from build123d import *

# Parameters (mm, degrees)
BOSS_EXTRUDE1_DEPTH = 20.5
SKETCH2_W           = 11
SKETCH2_H           = 11
CUT_EXTRUDE1_DEPTH  = 38.791732231
SKETCH3_W           = 30.25
SKETCH3_H           = 17.75
CUT_EXTRUDE2_DEPTH  = 0.5
CUT_EXTRUDE3_REACH  = 39.609
SKETCH4_W           = 27.25
SKETCH4_H           = 14.75
SKETCH5_W           = 2
SKETCH5_H           = 1.375
SKETCH5_W_2         = 1.375
SKETCH5_H_2         = 2
BOSS_EXTRUDE2_DEPTH = 0.75
SKETCH6_W           = 1.375
SKETCH6_H           = 2
SKETCH6_W_2         = 0.3
SKETCH6_W_3         = 2
SKETCH6_H_2         = 0.3
SKETCH6_H_3         = 1.375
BOSS_EXTRUDE3_DEPTH = 0.75
SKETCH7_W           = 8
SKETCH7_H           = 2.5
CUT_EXTRUDE4_DEPTH  = 38.609374164
CUT_EXTRUDE5_REACH  = 39.528
SKETCH8_W           = 1
SKETCH8_H           = 11


with BuildPart() as part:
    # Sketch1 → Boss-Extrude1 (new body)
    with BuildSketch(Plane(origin=(0, 0, 0), x_dir=(1, 0, 0), z_dir=(0, 1, 0))):
        with BuildLine():
            Line((-21.150314886, 2.25), (-22.947265174, 1.37195122))
            ThreePointArc((-22.947265174, 1.37195122), (-22.710349254, 0.704078714), (-22.63, 0))
            ThreePointArc((-22.63, 0), (-26.459078714, -3.044650746), (-28.562734826, 1.37195122))
            Line((-28.562734826, 1.37195122), (-30.359685114, 2.25))
            ThreePointArc((-30.359685114, 2.25), (-26.90968909, -4.993227223), (-20.63, 0))
            ThreePointArc((-20.63, 0), (-20.643812376, 0.376013393), (-20.685175052, 0.75))
            ThreePointArc((-20.685175052, 0.75), (-20.85994778, 1.517922517), (-21.150314886, 2.25))
        make_face()
        with BuildLine():
            Line((21.150314886, 2.25), (-21.150314886, 2.25))
            ThreePointArc((-21.150314886, 2.25), (-20.85994778, 1.517922517), (-20.685175052, 0.75))
            Line((-20.685175052, 0.75), (20.685175052, 0.75))
            ThreePointArc((20.685175052, 0.75), (20.85994778, 1.517922517), (21.150314886, 2.25))
        make_face()
        with BuildLine():
            Line((22.947265174, 1.37195122), (21.150314886, 2.25))
            ThreePointArc((21.150314886, 2.25), (20.85994778, 1.517922517), (20.685175052, 0.75))
            ThreePointArc((20.685175052, 0.75), (25.378986607, -5.111187624), (30.88, 0))
            ThreePointArc((30.88, 0), (30.748227223, 1.15468909), (30.359685114, 2.25))
            Line((30.359685114, 2.25), (28.562734826, 1.37195122))
            ThreePointArc((28.562734826, 1.37195122), (28.799650746, 0.704078714), (28.88, 0))
            ThreePointArc((28.88, 0), (25.050921286, -3.044650746), (22.947265174, 1.37195122))
        make_face()
        with BuildLine():
            Line((23.586331053, 2.25), (21.150314886, 2.25))
            Line((21.150314886, 2.25), (22.947265174, 1.37195122))
            ThreePointArc((22.947265174, 1.37195122), (23.22836369, 1.838949145), (23.586331053, 2.25))
        make_face()
        with BuildLine():
            Line((28.562734826, 1.37195122), (30.359685114, 2.25))
            Line((30.359685114, 2.25), (27.923668947, 2.25))
            ThreePointArc((27.923668947, 2.25), (28.28163631, 1.838949145), (28.562734826, 1.37195122))
        make_face()
        with BuildLine():
            ThreePointArc((-23.586331053, 2.25), (-23.22836369, 1.838949145), (-22.947265174, 1.37195122))
            Line((-22.947265174, 1.37195122), (-21.150314886, 2.25))
            Line((-21.150314886, 2.25), (-23.586331053, 2.25))
        make_face()
        with BuildLine():
            Line((-30.359685114, 2.25), (-28.562734826, 1.37195122))
            ThreePointArc((-28.562734826, 1.37195122), (-28.28163631, 1.838949145), (-27.923668947, 2.25))
            Line((-27.923668947, 2.25), (-30.359685114, 2.25))
        make_face()
    extrude(amount=BOSS_EXTRUDE1_DEPTH)

    # Sketch2 → Cut-Extrude1 (cut, through all)
    with BuildSketch(Plane(origin=(0, 0, -2.25), x_dir=(-1, 0, 0), z_dir=(0, 0, -1))):
        with Locations((-25.38, 10.25)):
            Rectangle(SKETCH2_W, SKETCH2_H)
        with Locations((25.38, 10.25)):
            Rectangle(SKETCH2_W, SKETCH2_H)
    extrude(amount=-CUT_EXTRUDE1_DEPTH, mode=Mode.SUBTRACT)

    # Sketch3 → Cut-Extrude2 (cut)
    with BuildSketch(Plane.XY.offset(-0.75)):
        with Locations((0, 10.25)):
            Rectangle(SKETCH3_W, SKETCH3_H)
    extrude(amount=-CUT_EXTRUDE2_DEPTH, mode=Mode.SUBTRACT)

    # Sketch4 → Cut-Extrude3 (cut, up to next)
    with BuildSketch(Plane.XY.offset(-1.25), mode=Mode.PRIVATE) as cut_extrude3_sk1:
        with Locations((0, 10.25)):
            Rectangle(SKETCH4_W, SKETCH4_H)
    cut_extrude3_tool1 = extrude(cut_extrude3_sk1.sketch, amount=-CUT_EXTRUDE3_REACH, mode=Mode.PRIVATE) & part.part
    add(cut_extrude3_tool1.solids().sort_by_distance((0, 10.25, -1.25))[0], mode=Mode.SUBTRACT)

    # Sketch5 → Boss-Extrude2 (add)
    with BuildSketch(Plane.XY.offset(-0.75)):
        with Locations((0, 19.8125)):
            Rectangle(SKETCH5_W, SKETCH5_H)
        with Locations((0, 0.6875)):
            Rectangle(SKETCH5_W, SKETCH5_H)
        with Locations((-15.8125, 10.25)):
            Rectangle(SKETCH5_W_2, SKETCH5_H_2)
        with Locations((15.8125, 10.25)):
            Rectangle(SKETCH5_W_2, SKETCH5_H_2)
    extrude(amount=BOSS_EXTRUDE2_DEPTH)

    # Sketch6 → Boss-Extrude3 (add)
    with BuildSketch(Plane.XY):
        with Locations((-15.8125, 10.25)):
            Rectangle(SKETCH6_W, SKETCH6_H)
        with Locations((-14.975, 10.25)):
            Rectangle(SKETCH6_W_2, SKETCH6_H)
        with Locations((0, 1.525)):
            Rectangle(SKETCH6_W_3, SKETCH6_H_2)
        with Locations((0, 0.6875)):
            Rectangle(SKETCH6_W_3, SKETCH6_H_3)
        with Locations((14.975, 10.25)):
            Rectangle(SKETCH6_W_2, SKETCH6_H)
        with Locations((15.8125, 10.25)):
            Rectangle(SKETCH6_W, SKETCH6_H)
        with Locations((0, 19.8125)):
            Rectangle(SKETCH6_W_3, SKETCH6_H_3)
        with Locations((0, 18.975)):
            Rectangle(SKETCH6_W_3, SKETCH6_H_2)
    extrude(amount=BOSS_EXTRUDE3_DEPTH)

    # Sketch7 → Cut-Extrude4 (cut, through all)
    with BuildSketch(Plane.XY.offset(-1.25)):
        with Locations((-11.125, 17.875)):
            Rectangle(SKETCH7_W, SKETCH7_H)
    extrude(amount=-CUT_EXTRUDE4_DEPTH, mode=Mode.SUBTRACT)

    # Sketch8 → Cut-Extrude5 (cut, up to next)
    with BuildSketch(Plane.XY.offset(-0.75), mode=Mode.PRIVATE) as cut_extrude5_sk1:
        with Locations((19.38, 10.25)):
            Rectangle(SKETCH8_W, SKETCH8_H)
    cut_extrude5_tool1 = extrude(cut_extrude5_sk1.sketch, amount=-CUT_EXTRUDE5_REACH, mode=Mode.PRIVATE) & part.part
    add(cut_extrude5_tool1.solids().sort_by_distance((19.38, 10.25, -0.75))[0], mode=Mode.SUBTRACT)


solid = part.part
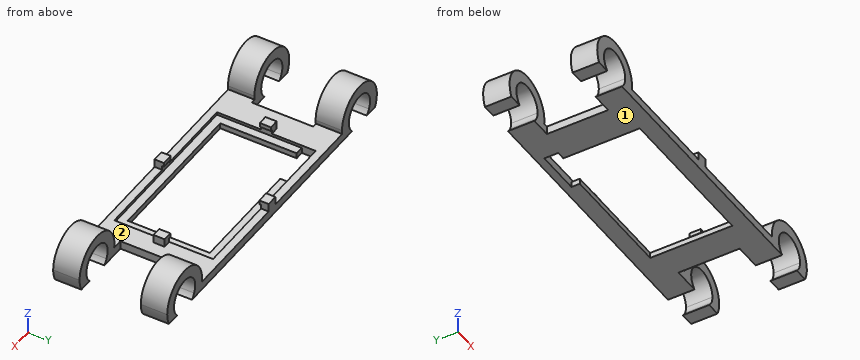
Check sheet for the modelled part. Datum: model origin and axes. Units: mm. Face numbers are marked on the shaded views. Round coordinates to 2 decimals unless told otherwise and drop trailing zeros. Write each loop counter-clockwise with the first axis right and the second up, starting at its lowest first coordinate (ties: lowest second). Pieces come first, ordered by that corner, then holes. Notation, with made-up numbers: (79, 0.25) -> (118, 0.25) arc R5 cw to (118, 5.25) -> close; hole circle Ø9 at (-10, 27.25). An arc over 180 degrees is marked (long way). Answer as CSV lines item,"result". Start each with the question number.
1) Section check D-D on z = 4.5. Enter the section's corners in (x, y), and give its area (3 significant figures).
2) Go/stop test with flat-tipped pins: P1, Ø1.3, axis at x = 15.5, y = 10, coming from the +Z side; P2, Ø0.8, axis at x = 16, z = 0, coming from the -Y side; P3, Ø1, axis at y = 2.5, z = -1.5, coming from the -X side. Record where each tip stops, or that it passes through.
3) Release check for a two-part mould opening along X. For the marked faces 1 and 2 record: pulls with the +X half, pulls with the -X half, needs draft (parallel to the pull), parting line crosses it, or undercut.
4) Material ranges on line 1 (Y direction, x = 26, z = 4); line 2 (X direction, y = 4.5, z = 2); line 3 (Y direction, x = -1, z = -1.5) (3 decimals), recorded low to high. Write a range as from..to.
5) Section check B-B on x = -11. Enter the section's corners in (y, z) (3 decimals).
6) Section check A-A on y = 14.5. Enter the section's corners in (x, z) (3 decimals).
7) Section check C-C on z = 1.5. State how many separate pieces and enclosed holes the cut face has, and give its area (3 significant figures).
Found:
1,outline,"(-28.21, 0) -> (-23.3, 0) -> (-23.3, 4.75) -> (-28.21, 4.75) -> close; (-28.21, 15.75) -> (-23.3, 15.75) -> (-23.3, 20.5) -> (-28.21, 20.5) -> close; (23.3, 0) -> (28.21, 0) -> (28.21, 4.75) -> (23.3, 4.75) -> close; (23.3, 15.75) -> (28.21, 15.75) -> (28.21, 20.5) -> (23.3, 20.5) -> close"
1,area,"93.2 mm^2"
2,P1,"stops at z = 0.75"
2,P2,"stops at y = 9.25"
2,P3,"stops at x = -30.78"
3,face 1,"needs draft"
3,face 2,"undercut"
4,line 1,"y = 0..4.75, 15.75..20.5"
4,line 2,"x = -30.47..-28.16, -23.35..-21.04, 21.04..23.35, 28.16..30.47"
4,line 3,"y = 0..2.875, 17.625..20.5"
5,outline,"(0, -2.25) -> (2.875, -2.25) -> (2.875, -1.25) -> (1.375, -1.25) -> (1.375, -0.75) -> (0, -0.75) -> close; (19.125, -2.25) -> (20.5, -2.25) -> (20.5, -0.75) -> (19.125, -0.75) -> close"
6,outline,"(-19.88, -2.25) -> (-13.625, -2.25) -> (-13.625, -1.25) -> (-15.125, -1.25) -> (-15.125, -0.75) -> (-19.88, -0.75) -> close; (13.625, -2.25) -> (18.88, -2.25) -> (18.88, -0.75) -> (15.125, -0.75) -> (15.125, -1.25) -> (13.625, -1.25) -> close"
7,separate pieces,"8"
7,enclosed holes,"0"
7,area,"82.0 mm^2"
